```python
from build123d import *

# Parameters (mm, degrees)
F0_W     = 80.772
F0_H     = 123.444
F0_R     = 3.175
F1_DEPTH = 3.175


# Not quite as in the source:
# - ends of sketch curves that miss each other by under 0.0002 mm in the source are joined


with BuildPart() as f1:
    # F0 (on Front) → F1 (new body)
    with BuildSketch(Plane.XZ):
        Rectangle(F0_W, F0_H)
        with BuildLine():
            ThreePointArc((-9.4932913315, -33.5419135021), (-16.889821539, -19.5719126303), (-9.4932913315, -5.6019117584))
            Line((-9.4932913315, -5.6019117584), (9.495647661, -5.6019126303))
            ThreePointArc((9.495647661, -5.6019126303), (16.892178461, -19.5719126303), (9.4956482536, -33.5419135021))
            Line((9.4956482536, -33.5419135021), (-9.4932913315, -33.5419135021))
        make_face(mode=Mode.SUBTRACT)
        with Locations((0.001178461, -0.0774126303)):
            Circle(F0_R, mode=Mode.SUBTRACT)
        with BuildLine():
            ThreePointArc((-9.4932913315, 5.4470864979), (-16.889821539, 19.4170873697), (-9.4932913315, 33.3870882416))
            Line((-9.4932913315, 33.3870882416), (9.495647661, 33.3870873697))
            ThreePointArc((9.495647661, 33.3870873697), (16.892178461, 19.4170873697), (9.4956482536, 5.4470864979))
            Line((9.4956482536, 5.4470864979), (-9.4932913315, 5.4470864979))
        make_face(mode=Mode.SUBTRACT)
    extrude(amount=F1_DEPTH)


solid = f1.part
```
Source: CAD feature listing. Evaluate the final solid. Frame: model axes, mm. A direction names the side the tool comes from. Coordinates: 2 decimals unless noted, no trailing zeros. Order: outer loops, then holes, each group sorted by start corner. A loop starts at its lowest first (then second) coordinate and runs counter-clockwise, first axis right, second up. Notation, with made-up numbers: M 53.5,-21 L 57.5,-21 A14 ccw 57.5,-12 Z; hole C 67,72 d4. An arc over 180 degrees is marked long. Write each question's results on one line, items separated by ' | '. Start each with the question number.
1) Section query C-C (y = -1.65). Return the cut outline in (x, z) (3 decimals), plus the area to 3 significant figures.
2) Section query A-A (x = -6). Return the cut outline in (y, z) (3 decimals), plus the area to 3 significant figures.
3) Section query B-B (z = -29). Return the cut outline in (x, y) (3 decimals).
4) Line query: line 1 (Z direction, x = 4, y = -2.95); line 2 (Z direction, x = -15, y = -2.5); line 3 (Z direction, x = 0.5, y = -2.2). Output: solid intervals per line, ascending. Write a range as from..to.
5) Draft query along Z for faces 3 (the face through (-1, -2, -61.722)), 4 (the face through (16.89, -1.57, 19.65)), 5 (the face through (8, 0, 1)). Return one class per face: released by +Z, released by -Z, zero draft, split by the parting line, or undercut.
6) Contact query for a flat-ended pin moving along its axis: pin 1 Ø2 at (x, z) = (-16.5, 16) entering from +Y. Output: stop coordinate, or through.
7) Access query for faces 1 (the face through (0, -2, 5.447)), 2 (the face through (-40.386, -2, -1)). Directions: +Z, -Z, +X, -X, +Y, -Y. A direction counts if a zero-diameter tool reaches every point of the face in a straight line with its end or side. Return the directions, or none.
8) Section query D-D (x = 15). Return the cut outline in (y, z) (3 decimals).
Answers:
1) outline: M -40.386,-61.722 L 40.386,-61.722 L 40.386,61.722 L -40.386,61.722 Z; hole M -9.493,-33.542 L 9.496,-33.542 A16.891 ccw 9.496,-5.602 L -9.493,-5.602 A16.891 ccw Z; hole M -9.493,5.447 L 9.496,5.447 A16.891 ccw 9.496,33.387 L -9.493,33.387 A16.891 ccw Z; hole C 0.001,-0.077 d6.35 | area: 8,300 mm^2
2) outline: M -3.175,-61.722 L 0,-61.722 L 0,-33.542 L -3.175,-33.542 Z; M -3.175,-5.602 L 0,-5.602 L 0,5.447 L -3.175,5.447 Z; M -3.175,33.387 L 0,33.387 L 0,61.722 L -3.175,61.722 Z | area: 215 mm^2
3) outline: M -40.386,-3.175 L -14.014,-3.175 L -14.014,0 L -40.386,0 Z; M 14.016,-3.175 L 40.386,-3.175 L 40.386,0 L 14.016,0 Z
4) line 1: z = -61.72..-33.54, -5.6..5.45, 33.39..61.72 | line 2: z = -61.72..-27.34, -11.81..11.65, 27.18..61.72 | line 3: z = -61.72..-33.54, -5.6..-3.21, 3.06..5.45, 33.39..61.72
5) face 3: released by -Z | face 4: undercut | face 5: zero draft
6) pin 1: stops at y = 0
7) face 1: +Y, -Y | face 2: +Z, -Z, -X, +Y, -Y
8) outline: M -3.175,-61.722 L 0,-61.722 L 0,-27.34 L -3.175,-27.34 Z; M -3.175,-11.804 L 0,-11.804 L 0,11.649 L -3.175,11.649 Z; M -3.175,27.185 L 0,27.185 L 0,61.722 L -3.175,61.722 Z
